from build123d import *

# Parameters (mm, degrees)
SKETCH1_R           = 14
SKETCH1_R_2         = 1.5
BOSS_EXTRUDE1_DEPTH = 5


with BuildPart() as part:
    # Sketch1 → Boss-Extrude1 (new body)
    with BuildSketch(Plane(origin=(0, 0, 0), x_dir=(1, 0, 0), z_dir=(0, 1, 0))):
        with BuildLine():
            Line((26.464466094, -43.035533906), (33.964466094, -35.535533906))
            ThreePointArc((33.964466094, -35.535533906), (37.5, -34.071067812), (41.035533906, -35.535533906))
            Line((41.035533906, -35.535533906), (48.535533906, -43.035533906))
            ThreePointArc((48.535533906, -43.035533906), (50.15765065, -44.119397663), (52.071067812, -44.5))
            Line((52.071067812, -44.5), (81, -44.5))
            ThreePointArc((81, -44.5), (88.071067812, -41.571067812), (91, -34.5))
            Line((91, -34.5), (91, 34.5))
            ThreePointArc((91, 34.5), (88.071067812, 41.571067812), (81, 44.5))
            Line((81, 44.5), (52.071067812, 44.5))
            ThreePointArc((52.071067812, 44.5), (50.15765065, 44.119397663), (48.535533906, 43.035533906))
            Line((48.535533906, 43.035533906), (41.035533906, 35.535533906))
            ThreePointArc((41.035533906, 35.535533906), (37.5, 34.071067812), (33.964466094, 35.535533906))
            Line((33.964466094, 35.535533906), (26.464466094, 43.035533906))
            ThreePointArc((26.464466094, 43.035533906), (24.84234935, 44.119397663), (22.928932188, 44.5))
            Line((22.928932188, 44.5), (-81, 44.5))
            ThreePointArc((-81, 44.5), (-88.071067812, 41.571067812), (-91, 34.5))
            Line((-91, 34.5), (-91, -34.5))
            ThreePointArc((-91, -34.5), (-88.071067812, -41.571067812), (-81, -44.5))
            Line((-81, -44.5), (22.928932188, -44.5))
            ThreePointArc((22.928932188, -44.5), (24.84234935, -44.119397663), (26.464466094, -43.035533906))
        make_face()
        with Locations((-8, 0)):
            Circle(SKETCH1_R, mode=Mode.SUBTRACT)
        with Locations((-30.273863607, 8.131727984)):
            Circle(SKETCH1_R_2, mode=Mode.SUBTRACT)
        with Locations((-16.131727984, 22.273863607)):
            Circle(SKETCH1_R_2, mode=Mode.SUBTRACT)
        with Locations((0.131727984, 22.273863607)):
            Circle(SKETCH1_R_2, mode=Mode.SUBTRACT)
        with Locations((14.273863607, 8.131727984)):
            Circle(SKETCH1_R_2, mode=Mode.SUBTRACT)
        with Locations((14.273863607, -8.131727984)):
            Circle(SKETCH1_R_2, mode=Mode.SUBTRACT)
        with Locations((0.131727984, -22.273863607)):
            Circle(SKETCH1_R_2, mode=Mode.SUBTRACT)
        with Locations((-16.131727984, -22.273863607)):
            Circle(SKETCH1_R_2, mode=Mode.SUBTRACT)
        with Locations((-30.273863607, -8.131727984)):
            Circle(SKETCH1_R_2, mode=Mode.SUBTRACT)
        with Locations((-75, -37.5)):
            Circle(SKETCH1_R_2, mode=Mode.SUBTRACT)
        with Locations((-57, -39.5)):
            Circle(SKETCH1_R_2, mode=Mode.SUBTRACT)
        with Locations((-18, -39.5)):
            Circle(SKETCH1_R_2, mode=Mode.SUBTRACT)
        with Locations((0, -37.5)):
            Circle(SKETCH1_R_2, mode=Mode.SUBTRACT)
        with Locations((18, -39.5)):
            Circle(SKETCH1_R_2, mode=Mode.SUBTRACT)
        with Locations((57, -39.5)):
            Circle(SKETCH1_R_2, mode=Mode.SUBTRACT)
        with Locations((75, -37.5)):
            Circle(SKETCH1_R_2, mode=Mode.SUBTRACT)
        with Locations((86, -18)):
            Circle(SKETCH1_R_2, mode=Mode.SUBTRACT)
        with Locations((86, 18)):
            Circle(SKETCH1_R_2, mode=Mode.SUBTRACT)
        with Locations((75, 37.5)):
            Circle(SKETCH1_R_2, mode=Mode.SUBTRACT)
        with Locations((57, 39.5)):
            Circle(SKETCH1_R_2, mode=Mode.SUBTRACT)
        with Locations((18, 39.5)):
            Circle(SKETCH1_R_2, mode=Mode.SUBTRACT)
        with Locations((0, 37.5)):
            Circle(SKETCH1_R_2, mode=Mode.SUBTRACT)
        with Locations((-18, 39.5)):
            Circle(SKETCH1_R_2, mode=Mode.SUBTRACT)
        with Locations((-57, 39.5)):
            Circle(SKETCH1_R_2, mode=Mode.SUBTRACT)
        with Locations((-75, 37.5)):
            Circle(SKETCH1_R_2, mode=Mode.SUBTRACT)
        with Locations((-86, 18)):
            Circle(SKETCH1_R_2, mode=Mode.SUBTRACT)
        with Locations((-86, -18)):
            Circle(SKETCH1_R_2, mode=Mode.SUBTRACT)
    extrude(amount=BOSS_EXTRUDE1_DEPTH)


solid = part.part
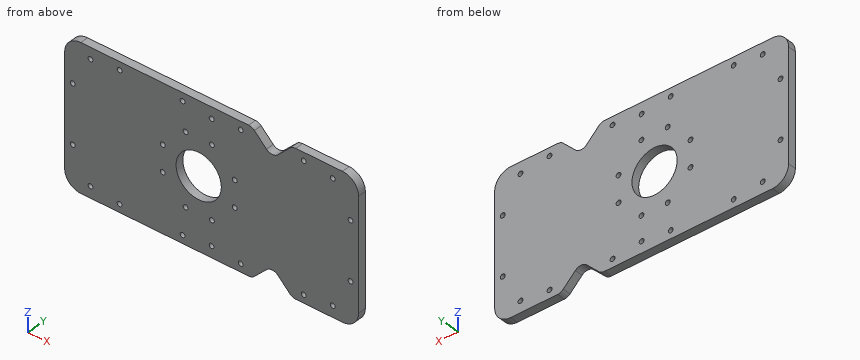
Part model, mm, in its own coordinate system. Round coordinates to 2 decimals unless told otherwise and drop trailing zeros. Loops run counter-clockwise (first coordinate to the right, second up) from the corner with the lowest first, then second, coordinate; pieces in that order, holes last. Notation, with made-up numbers: (86, 28.5) - (100, 28.5) arc R23 ccw to (100, 67.5) - close; hole circle Ø2 at (-11, 47). An arc over 180 degrees is marked (long way). Answer as a JSON object with one key per item and string values.
Item 1: Band-saw the part on A-A on x = -11.5. List the corners of the cut face in (y, z), plus the area to 3 significant figures.
Output:
{"outline": "(0, -44.5) - (5, -44.5) - (5, -13.56) - (0, -13.56) - close; (0, 13.56) - (5, 13.56) - (5, 44.5) - (0, 44.5) - close", "area": "309 mm2"}
Item 2: Wall check: L1, parallel to Z at x = 75, y = 4.15; L2, parallel to X at y = 2.45, z = -39.5; L3, parallel to X at y = 3.65, z = -37.5. Give the ranges that are in metal, low to high.
Output:
{"L1": "-44.5 to -39, -36 to 36, 39 to 44.5", "L2": "-89.66 to -58.5, -55.5 to -19.5, -16.5 to 16.5, 19.5 to 30, 45 to 55.5, 58.5 to 89.66", "L3": "-90.54 to -76.5, -73.5 to -1.5, 1.5 to 32, 43 to 73.5, 76.5 to 90.54"}
Item 3: Band-saw the part on B-B on x = 32. List the corners of the cut face in (y, z), plus the area to 3 significant figures.
Output:
{"outline": "(0, -37.5) - (5, -37.5) - (5, 37.5) - (0, 37.5) - close", "area": "375 mm2"}
Item 4: Band-saw the part on C-C on y = 2.3. State how many separate pieces and enclosed holes the cut face has, plus the area to 3 significant figures.
Output:
{"separate pieces": "1", "enclosed holes": "27", "area": "15,000 mm2"}
